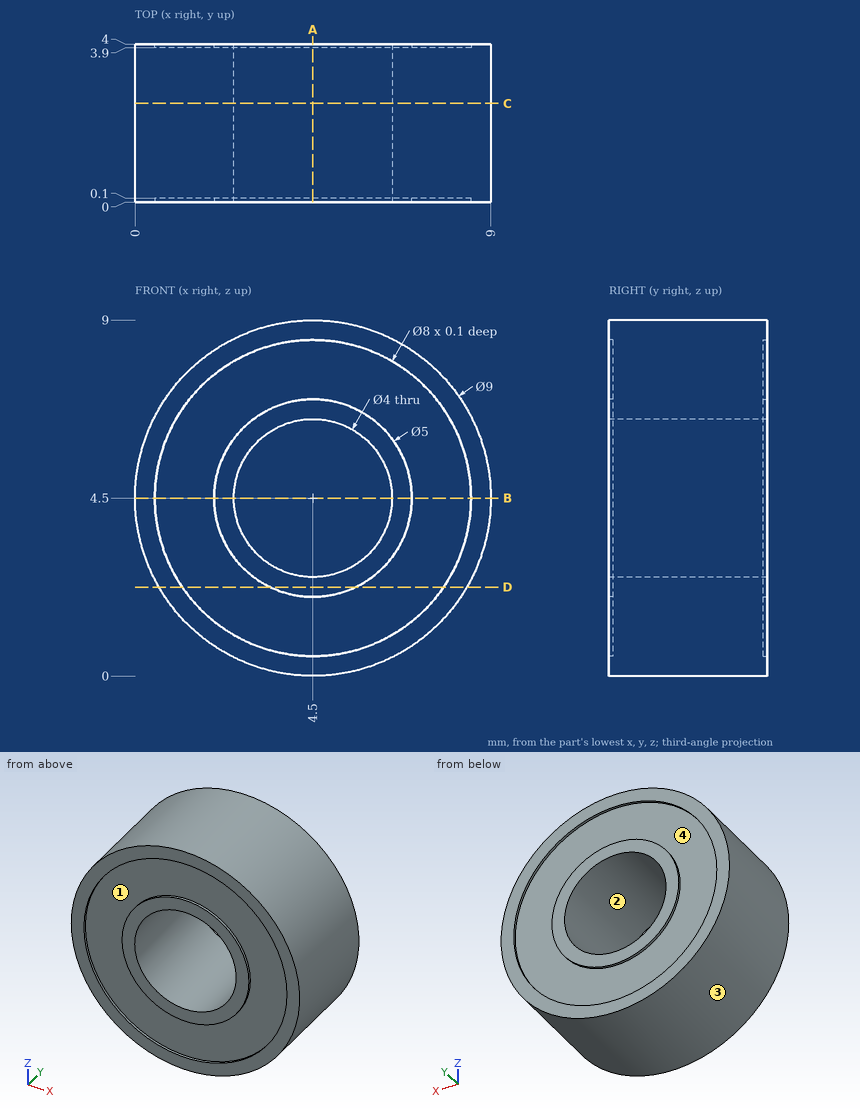
Geometry: see drawing. Coordinates: mm, zero at the bounding-box minimum. A direction names the side the tool comes from. Round coordinates to 2 decimals unless told otherwise and drop trailing zeros. Loops run counter-clockwise (first coordinate to the right, second up) from the corner with the lowest first, then second, coordinate; pieces in that order, holes last. Notation, with made-up numbers: M -5.5,-18 L 9.5,-18 A29 cw 9.5,2 Z; hole C 46,-2 d10. An arc over 180 degrees is marked long. Use a Markdown table: item, result. Add a question column.
1. Reachability of the marked faces 1 and 2 from +Z, -Z, +X, -X, +Y, -Y: full face, straight path, thin tool, end or side. Return the list, or none.
2. Section query C-C on y = 2.5. Return the cut outline in (x, z).
3. Mould query, pull axis X, two halves, no side actions, for the marked faces 3 and 4. Classes: pulls with the +X half, pulls with the -X half, needs draft (parallel to the pull), parting line crosses it, or undercut.
4. Contact query for flat-ended pins moving along their axis: P1, Ø1.5, axis at x = 4.5, z = 7.5, coming from the -Y side; P2, Ø2, axis at x = 6.5, y = 1.5, coming from the -Z side. Output: stop coordinate, or through.
5. Line query: line 1 (Z direction, x = 3.25, y = 2.8); line 2 (Z direction, x = 2.75, y = 2.15); line 3 (X direction, y = 0.55, z = 4.75). Output: solid intervals per line, ascending.
6. Section query D-D on z = 2.25. Return the cut outline in (x, y).
7. Section query A-A on x = 4.5. Return the cut outline in (y, z), then the cut area to 3 significant figures.
8. Section query B-B on z = 4.5. Return the cut outline in (x, y), then the cut area to 3 significant figures.
Reported:
| question | item | result |
|---|---|---|
| 1 | face 1 | -Y |
| 1 | face 2 | +Y, -Y |
| 2 | outline | C 4.5,4.5 d9; hole C 4.5,4.5 d4 |
| 3 | face 3 | parting line crosses it |
| 3 | face 4 | undercut |
| 4 | P1 | stops at y = 0 |
| 4 | P2 | stops at z = 0.11 |
| 5 | line 1 | z = 0.18 to 2.94, 6.06 to 8.82 |
| 5 | line 2 | z = 0.35 to 3.53, 5.47 to 8.65 |
| 5 | line 3 | x = 0.01 to 2.52, 6.48 to 8.99 |
| 6 | outline | M 0.6,0 L 1.19,0 L 1.19,0.1 L 3.41,0.1 L 3.41,0 L 5.59,0 L 5.59,0.1 L 7.81,0.1 L 7.81,0 L 8.4,0 L 8.4,4 L 7.81,4 L 7.81,3.9 L 5.59,3.9 L 5.59,4 L 3.41,4 L 3.41,3.9 L 1.19,3.9 L 1.19,4 L 0.6,4 Z |
| 7 | outline | M 0,0 L 4,0 L 4,0.5 L 3.9,0.5 L 3.9,2 L 4,2 L 4,2.5 L 0,2.5 L 0,2 L 0.1,2 L 0.1,0.5 L 0,0.5 Z; M 0,6.5 L 4,6.5 L 4,7 L 3.9,7 L 3.9,8.5 L 4,8.5 L 4,9 L 0,9 L 0,8.5 L 0.1,8.5 L 0.1,7 L 0,7 Z |
| 7 | area | 19.4 mm² |
| 8 | outline | M 0,0 L 0.5,0 L 0.5,0.1 L 2,0.1 L 2,0 L 2.5,0 L 2.5,4 L 2,4 L 2,3.9 L 0.5,3.9 L 0.5,4 L 0,4 Z; M 6.5,0 L 7,0 L 7,0.1 L 8.5,0.1 L 8.5,0 L 9,0 L 9,4 L 8.5,4 L 8.5,3.9 L 7,3.9 L 7,4 L 6.5,4 Z |
| 8 | area | 19.4 mm² |
